The listing builds one solid part. Answer for the finished solid, in the listing's coordinates (mm). Face numbers are marked on the shaded views. A direction names the side the tool comes from. Give positions to 0.01 mm unless a question says otherwise; leave off trailing zeros. Write each loop counter-clockwise with the first axis right and the second up, starting at its lowest first coordinate (ties: lowest second). Pieces come first, ordered by that corner, then holes.
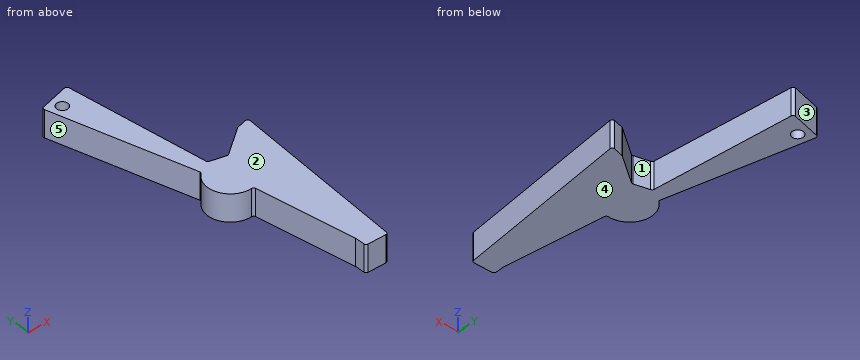
```python
from build123d import *

# Parameters (mm, degrees)
BOSS_EXTRUDE1_DEPTH = 12
SKETCH2_R           = 2.5
CUT_EXTRUDE1_DEPTH  = 139.979288596
FILLET1_R           = 1


with BuildPart() as part:
    # Sketch1 → Boss-Extrude1 (new body)
    with BuildSketch(Plane.XY):
        with BuildLine():
            Line((0, 0), (-14.488887394, -3.882285677))
            Line((-14.488887394, -3.882285677), (2.334350537, -66.667464385))
            ThreePointArc((2.334350537, -66.667464385), (-0.8237016, -78.663286709), (10.120361434, -84.502852689))
            Line((10.120361434, -84.502852689), (17.159912361, -128.948828016))
            Line((17.159912361, -128.948828016), (17.159912361, -134.180494133))
            Line((17.159912361, -134.180494133), (27.159912361, -134.180494133))
            Line((27.159912361, -134.180494133), (34.159005443, -54.180494133))
            Line((34.159005443, -54.180494133), (28.363450485, -55.733408403))
            Line((28.363450485, -55.733408403), (15.585282325, -65.362448774))
            Line((15.585282325, -65.362448774), (7.799637978, -63.522953705))
            Line((7.799637978, -63.522953705), (0, 0))
        make_face()
    extrude(amount=BOSS_EXTRUDE1_DEPTH)

    # Sketch2 → Cut-Extrude1 (cut, through all)
    with BuildSketch(Plane.XY.offset(12)):
        with Locations((-8.365163037, -7.417819582)):
            Circle(SKETCH2_R)
    extrude(amount=-CUT_EXTRUDE1_DEPTH, mode=Mode.SUBTRACT)

    # Fillet1
    fillet1_edges = [part.edges().sort_by_distance(p)[0] for p in [
        (7.799637978, -63.522953705, 6),
        (15.585282325, -65.362448774, 6),
        (28.363450485, -55.733408403, 6),
        (34.159005443, -54.180494133, 6),
        (27.159912361, -134.180494133, 6),
        (17.159912361, -134.180494133, 6),
        (10.120361434, -84.502852689, 6),
        (2.334350537, -66.667464385, 6),
        (-14.488887394, -3.882285677, 6),
        (0, 0, 6),
    ]]
    fillet(fillet1_edges, radius=FILLET1_R)


solid = part.part
```
Item 1: Which of the six approach directions +Z, -Z, +X, -X, +Y, -Y give full straight-line access (tool end or side, diameter ignored) to the marked faces 4 and 5?
Conclusion:
face 4: -Z, +X, -X, +Y, -Y
face 5: +Z, -Z, -X
Item 2: Consider probe 1 along X at (y, z) = (-60, 10.75); probe 2 along X at (y, z) = (-101, 5.75); probe 3 along X at (y, z) = (-41, 6). Determine where each line is inside the solid, lowest interval first.
Conclusion:
probe 1: x = 0.55 to 7.37, 22.7 to 33.65
probe 2: x = 12.73 to 30.06
probe 3: x = -4.54 to 5.03
Item 3: A cutting plane is placed at B-B, the plane y = -102. Give the vertices of the cut face in (x, z), plus the area to 3 significant figures.
Conclusion:
outline: (12.89, 0) - (29.98, 0) - (29.98, 12) - (12.89, 12) - close
area: 205 mm2
Item 4: A cutting plane is placed at A-A, the plane z = 3.5. Give the vertices of the cut face in (x, y), plus the area to 3 significant figures.
Conclusion:
outline: (-14.23, -4.85) - (2.17, -66.04) arc R1 cw to (1.85, -67.06) arc R10 ccw to (9.2, -84.63) arc R1 cw to (10.27, -85.47) - (17.16, -128.95) - (17.16, -133.18) arc R1 ccw to (18.16, -134.18) - (26.24, -134.18) arc R1 ccw to (27.24, -133.27) - (34.03, -55.6) arc R1 ccw to (32.78, -54.55) - (28.55, -55.68) arc R1 ccw to (28.21, -55.85) - (15.96, -65.08) arc R1 cw to (15.13, -65.25) - (8.48, -63.68) arc R1 cw to (7.71, -62.83) - (0.14, -1.14) arc R1 ccw to (-1.11, -0.3) - (-13.52, -3.62) arc R1 ccw to start; hole circle Ø5 at (-8.37, -7.42)
area: 2,160 mm2
Item 5: A cutting plane is placed at C-C, the plane x = 13.5. Give the vertices of the cut face in (y, z), plus the area to 3 significant figures.
Conclusion:
outline: (-105.84, 0) - (-64.87, 0) - (-64.87, 12) - (-105.84, 12) - close
area: 492 mm2
Item 6: Determine the mould class of the marked faces 1, 2 and 3 for opening direction X: pulls with the +X half, pulls with the -X half, needs draft (parallel to the pull), parting line crosses it, or undercut.
Conclusion:
face 1: undercut
face 2: needs draft
face 3: pulls with the -X half
Item 7: Each of these flat-tipped pins is pushed along its axis until it touches: P1, Ø4, axis at y = -30.5, z = 5.5, coming from the -X side; P2, Ø6, axis at y = -19, z = 4.5, coming from the -X side; P3, Ø6, axis at y = -64, z = 2.5, coming from the +X side. Where does it stop, or does it pass through?
Conclusion:
P1: stops at x = -7.89
P2: stops at x = -11.24
P3: stops at x = 33.56
